Read the model definition and answer for the solid it produces. Units are mm, in the model's axes. A direction names the side the tool comes from. Coordinates: 2 decimals unless noted, no trailing zeros. Order: outer loops, then holes, each group sorted by start corner. A loop starts at its lowest first (then second) coordinate and runs counter-clockwise, first axis right, second up.
from build123d import *

# Parameters (mm, degrees)
F1_DEPTH  = 9.017
F2_R      = 7.9375
F3_DEPTH  = 0.2794
F4_R      = 6.00075
F5_DEPTH  = 22.86
F6_R      = 4.76123
F7_DEPTH  = 50.0634
F8_R      = 4.49961
F9_DEPTH  = 69.85
F10_R     = 3.9624
F11_DEPTH = 92.075
F15_W     = 1.1811
F15_H     = 2.286
F17_R     = 7.9375
F18_DEPTH = 0.254
F19_R     = 3.95097
F20_DEPTH = 25.4
F21_R     = 1.7526
F22_DEPTH = 9.525


# Not quite as in the source:
# - a fillet or chamfer that OpenCascade refuses, or shapes differently, is made with other operations: its cross-section is extruded or revolved along the edge and cut away or added
# - a feature of the source that left no trace in its solid (it failed there, or was rolled back) is left out


with BuildPart() as f1:
    # F0 (on Front) → F1 (new body)
    with BuildSketch(Plane.XZ):
        Polygon((7.9375, 20.32), (0, 20.32), (-7.9375, 20.32), (-7.9375, 0), (-7.9375, -20.32), (0, -20.32), (7.9375, -20.32), (7.9375, 0), align=None)
    extrude(amount=F1_DEPTH)

    # F2 (on face) → F3 (join)
    with BuildSketch(Plane.XZ.offset(9.017)):
        Circle(F2_R)
    extrude(amount=F3_DEPTH)

    # F4 (on face) → F5 (join)
    with BuildSketch(Plane.XZ.offset(9.2964)):
        Circle(F4_R)
    extrude(amount=F5_DEPTH)

    # F6 (on face) → F7 (join)
    with BuildSketch(Plane.XZ.offset(9.2964)):
        Circle(F6_R)
    extrude(amount=F7_DEPTH)

    # F8 (on face) → F9 (join)
    with BuildSketch(Plane.XZ.offset(9.2964)):
        Circle(F8_R)
    extrude(amount=F9_DEPTH)

    # F10 (on face) → F11 (join)
    with BuildSketch(Plane.XZ.offset(9.2964)):
        Circle(F10_R)
    extrude(amount=F11_DEPTH)

    # F14: fillet of radius 1.016 on 3 edges, made by hand

    # F14_s1 → F14_t2 (revolve)
    with BuildSketch(Plane.XY):
        with BuildLine():
            ThreePointArc((5.77723, -32.1564), (5.0588095103, -32.4539795103), (4.76123, -33.1724))
            Line((4.76123, -33.1724), (4.76123, -32.1564))
            Line((4.76123, -32.1564), (5.77723, -32.1564))
        make_face()
    revolve(axis=Axis((0, -32.1564, 0), (0, 1, 0)))

    # F14_s3 → F14_t4 (revolve)
    with BuildSketch(Plane.XY):
        with BuildLine():
            ThreePointArc((4.76123, -59.3598), (4.5672677411, -59.675805019), (4.49961, -60.0403636014))
            Line((4.49961, -60.0403636014), (4.49961, -59.3598))
            Line((4.49961, -59.3598), (4.76123, -59.3598))
        make_face()
    revolve(axis=Axis((0, -59.3598, 0), (0, 1, 0)))

    # F14_s5 → F14_t6 (revolve)
    with BuildSketch(Plane.XY):
        with BuildLine():
            ThreePointArc((4.49961, -79.1464), (4.1069911866, -79.5201107955), (3.9624, -80.042511676))
            Line((3.9624, -80.042511676), (3.9624, -79.1464))
            Line((3.9624, -79.1464), (4.49961, -79.1464))
        make_face()
    revolve(axis=Axis((0, -79.1464, 0), (0, 1, 0)))

    # F15 (on Right) → F16 (revolve, cut)
    with BuildSketch(Plane.YZ):
        with Locations((-21.38045, 4.85775)):
            Rectangle(F15_W, F15_H)
    revolve(axis=Axis((0, -21.971, 4.85775), (0, 0, -1)), mode=Mode.SUBTRACT)

    # F17 (on face) → F18 (join)
    with BuildSketch(Plane(origin=(0, 0, 0), x_dir=(-1, 0, 0), z_dir=(0, 1, 0))):
        with Locations((0, 12.3825)):
            Circle(F17_R)
    extrude(amount=F18_DEPTH)

    # F19 (on face) → F20 (cut)
    with BuildSketch(Plane(origin=(0, 0.254, 0), x_dir=(-1, 0, 0), z_dir=(0, 1, 0))):
        with Locations((0, 12.3825)):
            Circle(F19_R)
    extrude(amount=-F20_DEPTH, mode=Mode.SUBTRACT)

    # F21 (on face) → F22 (cut)
    with BuildSketch(Plane(origin=(0, 0, -20.32), x_dir=(1, 0, 0), z_dir=(0, 0, -1))):
        with Locations((4.445, 4.5085)):
            Circle(F21_R)
        with Locations((-4.445, 4.5085)):
            Circle(F21_R)
    extrude(amount=-F22_DEPTH, mode=Mode.SUBTRACT)


solid = f1.part
Q1. Which of the six approach directions +Z, -Z, +X, -X, +Y, -Y give full straight-line access (tool end or side, diameter ignored) to faces 1 (the cylindrical face through (-3.503, -5.986, -15.624)), 2 (the flat face through (-2, -9.296, 6)), 3 (the flat face through (6, 0, 19)), 4 (the flat face through (0, -22, 3.715))?
Q2. Each of these flat-tipped pins is pushed along its axis until it touches: P1, Ø5, axis at y = -24.5, z = -7, coming from the -X side; P2, Ø8, axis at y = -80, z = 4, coming from the -X side; P3, Ø5, axis at x = -0.5, z = -11, coming from the -Y side. Where does it stop, or does it pass through?
Q3. Determine the mould class of faces 5 (the flat face through (-4, -9.017, 15)), 6 (the flat face through (0, -4, -20.32)), 7 (the cylindrical face through (-0.5, -20.9, 4.9)) for opening direction Y: +Y half, -Y half, draft (parallel to the pull), parting line (faces both ways), or undercut.
Q4. The part is cut by section B-B, the plane y = -89.5. Determine the outline of the cut face in (x, z).
Q5. Straight lines are drawn through the part: L1, parallel to Z at x = 0, y = -4.25; L2, parallel to Y at x = 0, z = -9.5; L3, parallel to Y at x = 2, z = -7. For each, find the intervals that lie inside material, in ascending order.
Q6. The part is cut by section A-A, the plane y = -41.5. Determine the outline of the cut face in (x, z), then the cut area to 3 significant figures.
Computed values:
1. face 1: -Z
1. face 2: -Y
1. face 3: +Z, +X, +Y
1. face 4: +Z
2. P1: stops at x = -3.97
2. P2: stops at x = -4.5
2. P3: stops at y = -9.02
3. face 5: -Y half
3. face 6: draft
3. face 7: undercut
4. outline: circle Ø7.92 at (0, 0)
5. L1: z = -20.32 to 8.43, 16.33 to 20.32
5. L2: y = -9.02 to 0
5. L3: y = -9.3 to 0
6. outline: circle Ø9.52 at (0, 0)
6. area: 71.2 mm2
